Read the model definition and answer for the solid it produces. Units are mm, in the model's axes. A direction names the side the tool comes from. Coordinates: 2 decimals unless noted, no trailing zeros. Write each loop counter-clockwise with the first axis right and the second up, starting at its lowest first coordinate (ties: lowest second). Pieces come first, ordered by that corner, then holes. Notation, with made-up numbers: M 21,66 L 30,66 A16 cw 30,96 Z; hole C 83,-28 d7. An arc over 180 degrees is marked long. Use a Markdown table: item, result. Add a question column.
Autodesk Inventor part; units mm, degrees
ref_plane "作業平面1" through (15, 0, 0) normal (1, 0, 0) x (0, 1, 0)
ref_plane "作業平面2" through (-15, 0, 0) normal (1, 0, 0) x (0, 1, 0)
ref_plane "作業平面3" through (0, 15, 0) normal (0, 1, 0) x (-1, 0, 0)
sketch "スケッチ2" plane through (0, 0, 0) normal (0, 0, 1) x (1, 0, 0)
  circle A0 centre (0, 0) radius 15.8
  dimension "d0" = 31.6
extrude "押し出し1" add sketch "スケッチ2" against normal blind 10
sketch "スケッチ13" plane through (0, 0, 0) normal (0, 0, 1) x (1, 0, 0)
  circle A0 centre (0, -3) radius 1.7
  circle A1 centre (-10, -6) radius 1.7
  circle A2 centre (10, -6) radius 1.7
  line L0 (0, 0) -> (0, 17.9574) construction
  dimension "d90" = 3.4
  dimension "d91" = 3.4
  dimension "d92" = 3.4
  dimension "d93" = 3
  dimension "d94" = 6
  dimension "d95" = 10
extrude "押し出し11" cut sketch "スケッチ13" against normal through all
sketch "スケッチ14" plane through (0, 0, 0) normal (0, 0, 1) x (1, 0, 0)
  circle A0 centre (0, -11.5) radius 2.15
  circle A1 centre (9.9593, 5.75) radius 2.15
  circle A2 centre (-9.9593, 5.75) radius 2.15
  point P0 (0, 0)
  dimension "d98" = 4.3
  dimension "d99" = 11.5
  dimension "d102" = 360
extrude "押し出し12" cut sketch "スケッチ14" against normal blind 1
ref_plane "作業平面1" through (15, 0, 0) normal (1, 0, 0) x (0, 1, 0)
ref_plane "作業平面2" through (-15, 0, 0) normal (1, 0, 0) x (0, 1, 0)
ref_plane "作業平面3" through (0, 15, 0) normal (0, 1, 0) x (-1, 0, 0)
ref_plane "作業平面4" through (0, -15, 0) normal (0, 1, 0) x (-1, 0, 0)
sketch "スケッチ22" plane through (0, 0, -10) normal (0, 0, -1) x (-1, 0, 0)
  arc A0 (4.5, -11.5) -> (-4.5, -11.5) centre (0, -11.5) ccw
  line L0 (-4.5, -11.5) -> (-4.5, -15.8)
  line L1 (-4.5, -15.8) -> (4.5, -15.8)
  line L2 (4.5, -15.8) -> (4.5, -11.5)
  arc A1 (7.7093, 9.6471) -> (12.2093, 1.8529) centre (9.9593, 5.75) ccw
  line L3 (11.4332, 11.7971) -> (7.7093, 9.6471)
  line L4 (15.9332, 4.0029) -> (11.4332, 11.7971)
  line L5 (12.2093, 1.8529) -> (15.9332, 4.0029)
  arc A2 (-12.2093, 1.8529) -> (-7.7093, 9.6471) centre (-9.9593, 5.75) ccw
  line L6 (-15.9332, 4.0029) -> (-12.2093, 1.8529)
  line L7 (-11.4332, 11.7971) -> (-15.9332, 4.0029)
  line L8 (-7.7093, 9.6471) -> (-11.4332, 11.7971)
  point P0 (0, 0)
  dimension "d129" = 4.5
  dimension "d132" = 360
extrude "押し出し17" cut sketch "スケッチ22" against normal blind 9
sketch "スケッチ23" plane through (15, 0, 0) normal (1, 0, 0) x (0, 1, 0)
  point P0 (0, 0)
sketch "スケッチ24" plane through (0, 0, -10) normal (0, 0, -1) x (-1, 0, 0)
  circle A0 centre (0, 0) radius 15.8
  circle A1 centre (0, 0) radius 15
  dimension "d136" = 30
extrude "押し出し18" cut sketch "スケッチ24" against normal blind 9
sketch "スケッチ25" plane through (15, 0, 0) normal (1, 0, 0) x (0, 1, 0)
  circle A0 centre (0, -6) radius 1
  line L0 (-14.3091, -10) -> (3.2574, -10)
  line L1 (15.8, -1) -> (-15.8, -1)
  point P0 (0, 0)
  dimension "d139" = 2
  dimension "d141" = 5
sketch "スケッチ27" plane through (0, 15, 0) normal (0, 1, 0) x (-1, 0, 0)
  circle A0 centre (0, -6) radius 1
  line L0 (15.8, -1) -> (-15.8, -1)
  point P0 (0, 0)
  dimension "d142" = 2
  dimension "d143" = 5
sketch "スケッチ28" plane through (-15, 0, 0) normal (1, 0, 0) x (0, 1, 0)
  circle A0 centre (0, -6) radius 1
  line L0 (15.8, -1) -> (-15.8, -1)
  point P0 (0, 0)
  dimension "d144" = 2
  dimension "d145" = 5
extrude "押し出し19" cut sketch "スケッチ25" against normal blind 6
extrude "押し出し20" cut sketch "スケッチ27" against normal blind 6
extrude "押し出し21" cut sketch "スケッチ28" along normal blind 6
thread "ねじ9"
thread "ねじ10"
thread "ねじ11"
properties part number "B_pipe_cylinder_5_1_1" material "ステンレス鋼 440C"
Item 1: Find section C-C on y = 12. Give the vertices of the cut face in (x, z).
Item 2: Find section D-D on x = -3.5. Give the vertices of the cut face in (y, z).
Item 3: Determine the mould class of faces 1 (the cylindrical face through (0, 12, -5)), 2 (the cylindrical face through (-0.221, -1.314, -4.93)), 3 (the flat face through (9, 0, -6)) for opening direction Z: pulls with the +Z half, pulls with the -Z half, needs draft (parallel to the pull), parting line crosses it, or undercut.
Item 4: For faces 4 (the flat face through (0, 9, -6)), 5 (the flat face through (-8.943, 10.359, -5.563)), 6 (the flat face through (8.91, 10.34, -5.56)), 7 (the cylindrical face through (0, -7, -6)), 8 (the cylindrical face through (6.113, 3.415, -5.563)), determine the directions among +Z, -Z, +X, -X, +Y, -Y from which every point of the face is accessible in a straight line to the end or side of a thin tool.
Item 5: Each of these flat-tipped pins is pushed along its axis until it touches: pin 1 (1.2 mm diameter, centred on y = 0, z = -6, fed in from -X); pin 2 (1 mm diameter, centred on y = 0, z = -6, fed in from +X); pin 3 (5 mm diameter, centred on x = 0, y = -11.5, fed in from -Z). Where does it stop, or does it pass through?
Item 6: Find section B-B on y = -11. Give the vertices of the cut face in (x, z).
Item 7: Consider probe 1 along Y at (x, z) = (0, -0.5); probe 2 along Y at (x, z) = (10, -6.75); probe 3 along Z at (x, y) = (0, 13). Determine where each line is inside the solid, lowest interval first.
Item 8: Find section A-A on z = -7.75. Give the vertices of the cut face in (x, y).
Geometry says:
| question | item | result |
|---|---|---|
| 1 | outline | M -10.28,-1 L -9,-1 L -9,-10 L 9,-10 L 9,-1 L 10.28,-1 L 10.28,0 L -10.28,0 Z; hole C 0,-6 d2 |
| 2 | outline | M -15.41,-1 L -8.67,-1 L -8.67,-10 L 14.59,-10 L 14.59,-1 L 15.41,-1 L 15.41,0 L -15.41,0 Z |
| 3 | face 1 | undercut |
| 3 | face 2 | needs draft |
| 3 | face 3 | undercut |
| 4 | face 4 | +Y |
| 4 | face 5 | -Z, -X |
| 4 | face 6 | -Z, +X |
| 4 | face 7 | -Z, -Y |
| 4 | face 8 | -Z |
| 5 | pin 1 | stops at x = -9 |
| 5 | pin 2 | stops at x = 9 |
| 5 | pin 3 | stops at z = -1 |
| 6 | outline | M -11.34,-1 L -10.2,-1 L -10.2,-10 L -4.47,-10 L -4.47,-1 L -2.09,-1 L -2.09,0 L -11.34,0 Z; M 2.09,-1 L 4.47,-1 L 4.47,-10 L 10.2,-10 L 10.2,-1 L 11.34,-1 L 11.34,0 L 2.09,0 Z |
| 7 | probe 1 | y = -15.8 to -13.65, -9.35 to -4.7, -1.3 to 15.8 |
| 7 | probe 2 | y = -11.18 to -7.7, -4.3 to -0.66, 0.66 to 1.25, 10.97 to 11.18 |
| 7 | probe 3 | z = -10 to -7, -5 to 0 |
| 8 | outline | M -14.64,3.26 A15 ccw -4.5,-14.31 L -4.5,-11.5 A4.5 cw 4.5,-11.5 L 4.5,-14.31 A15 ccw 14.64,3.26 L 12.21,1.85 A4.5 cw 7.71,9.65 L 10.14,11.05 A15 ccw -10.14,11.05 L -7.71,9.65 A4.5 cw -12.21,1.85 Z; hole C -10,-6 d3.4; hole C 0,-3 d3.4; hole C 10,-6 d3.4 |
